Verification items for the finished model (mm, model axes). Face numbers are marked on the shaded views. A direction names the side the tool comes from. Give positions to 0.01 mm unless a question says otherwise; leave off trailing zeros. Write each loop counter-clockwise with the first axis right and the second up, starting at its lowest first coordinate (ties: lowest second). Pieces come first, ordered by that corner, then holes. Notation, with made-up numbers: M -15.5,15.25 L 17.5,15.25 A9 ccw 17.5,27.25 Z; hole C -24.5,62 d10. An arc over 180 degrees is marked long. Answer as a JSON object with one key per item and string values.
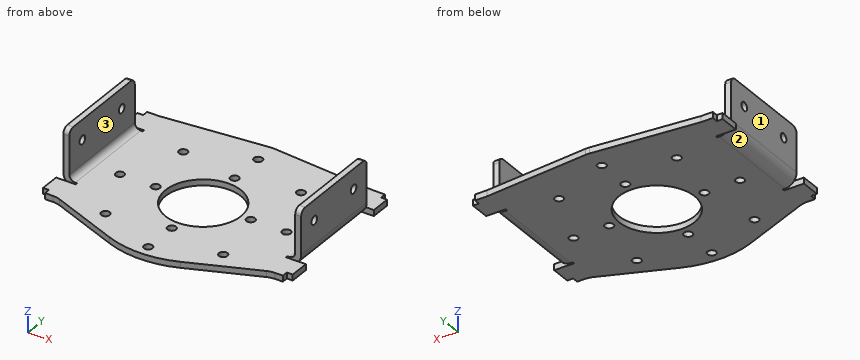
```python
from build123d import *

# Parameters (mm, degrees)
SKETCH1_R                = 19.05
SKETCH1_R_2              = 1
BASE_FLANGE1_DEPTH       = 3
UP_DEPTH                 = 50
UP_START                 = -3
UP_PROFILE_W             = 50
UP_PROFILE_H             = 22
UP_PROFILE_R             = 1
UP_FLAT_DEPTH            = 3
M4_CLEARANCE_HOLE1_D     = 4.3
M4_CLEARANCE_HOLE1_DEPTH = 136
M4_CLEARANCE_HOLE1_TIP   = 1.291850331
M4_CLEARANCE_HOLE2_D     = 4.3
M4_CLEARANCE_HOLE2_DEPTH = 136
M4_CLEARANCE_HOLE2_TIP   = 1.291850331
FILLET1_R                = 10
FILLET2_R                = 3


# Sheet-metal steps are written as plain solids
with BuildPart() as part:
    # Sketch1 → Base-Flange1 (new body)
    with BuildSketch(Plane.XY):
        with BuildLine():
            Line((-54, -30), (-17.930398419, -44.525282846))
            ThreePointArc((-17.930398419, -44.525282846), (0, -48), (17.930398419, -44.525282846))
            Line((17.930398419, -44.525282846), (54, -30))
            Line((54, -30), (60, -30))
            Line((60, -30), (60, -27))
            Line((60, -27), (63, -27))
            Line((63, -27), (63, -17))
            Line((63, -17), (53, -17))
            Line((53, -17), (53, -16))
            Line((53, -16), (54, -16))
            Line((54, -16), (54, 34))
            Line((54, 34), (53, 34))
            Line((53, 34), (53, 35))
            Line((53, 35), (63, 35))
            Line((63, 35), (63, 45))
            Line((63, 45), (60, 45))
            Line((60, 45), (60, 48))
            Line((60, 48), (54, 48))
            Line((54, 48), (0, 53))
            Line((0, 53), (-54, 48))
            Line((-54, 48), (-60, 48))
            Line((-60, 48), (-60, 45))
            Line((-60, 45), (-63, 45))
            Line((-63, 45), (-63, 35))
            Line((-63, 35), (-53, 35))
            Line((-53, 35), (-53, 34))
            Line((-53, 34), (-54, 34))
            Line((-54, 34), (-54, -16))
            Line((-54, -16), (-53, -16))
            Line((-53, -16), (-53, -17))
            Line((-53, -17), (-63, -17))
            Line((-63, -17), (-63, -27))
            Line((-63, -27), (-60, -27))
            Line((-60, -27), (-60, -30))
            Line((-60, -30), (-54, -30))
        make_face()
        Circle(SKETCH1_R, mode=Mode.SUBTRACT)
        with Locations((0, 24)):
            Circle(SKETCH1_R_2, mode=Mode.SUBTRACT)
        with Locations((0, -42)):
            Circle(SKETCH1_R_2, mode=Mode.SUBTRACT)
        with Locations((-29.69848481, -29.69848481)):
            Circle(SKETCH1_R_2, mode=Mode.SUBTRACT)
        with Locations((-42, 0)):
            Circle(SKETCH1_R_2, mode=Mode.SUBTRACT)
        with Locations((-29.69848481, 29.69848481)):
            Circle(SKETCH1_R_2, mode=Mode.SUBTRACT)
        with Locations((0, 42)):
            Circle(SKETCH1_R_2, mode=Mode.SUBTRACT)
        with Locations((29.69848481, 29.69848481)):
            Circle(SKETCH1_R_2, mode=Mode.SUBTRACT)
        with Locations((42, 0)):
            Circle(SKETCH1_R_2, mode=Mode.SUBTRACT)
        with Locations((29.69848481, -29.69848481)):
            Circle(SKETCH1_R_2, mode=Mode.SUBTRACT)
        with Locations((24, 0)):
            Circle(SKETCH1_R_2, mode=Mode.SUBTRACT)
        with Locations((0, -24)):
            Circle(SKETCH1_R_2, mode=Mode.SUBTRACT)
        with Locations((-24, 0)):
            Circle(SKETCH1_R_2, mode=Mode.SUBTRACT)
    extrude(amount=-BASE_FLANGE1_DEPTH)

    # UP bend section (across the edge) → UP (add)
    with BuildSketch(Plane(origin=(-57, 34, 0), x_dir=(1, 0, 0), z_dir=(0, -1, 0))):
        with BuildLine():
            Line((-3, 3), (0, 3))
            ThreePointArc((0, 3), (0.878679656, 0.878679656), (3, 0))
            Line((3, 0), (3, -3))
            ThreePointArc((3, -3), (-1.242640687, -1.242640687), (-3, 3))
        make_face()
    up = extrude(amount=UP_DEPTH)

    # UP profile (on flange) → UP flat (add)
    with BuildSketch(Plane.YZ.offset(-57).offset(UP_START)):
        with Locations((9, 14)):
            Rectangle(UP_PROFILE_W, UP_PROFILE_H)
        with Locations((-6, 15)):
            Circle(UP_PROFILE_R, mode=Mode.SUBTRACT)
        with Locations((24, 15)):
            Circle(UP_PROFILE_R, mode=Mode.SUBTRACT)
    up_flat = extrude(amount=UP_FLAT_DEPTH)

    # Mirror1: UP, UP flat across plane
    add(up.mirror(Plane(origin=(0, 0, 0), x_dir=(0, 0, 1), z_dir=(1, 0, 0))))
    add(up_flat.mirror(Plane(origin=(0, 0, 0), x_dir=(0, 0, 1), z_dir=(1, 0, 0))))

    # M4 Clearance Hole1
    with Locations(Plane.XY):
        with Locations((0, 24), (24, 0), (-24, 0), (0, -24), (0, -42), (29.69848481, -29.69848481), (42, 0), (29.69848481, 29.69848481), (0, 42), (-29.69848481, 29.69848481), (-42, 0), (-29.69848481, -29.69848481)):
            Hole(M4_CLEARANCE_HOLE1_D / 2, depth=M4_CLEARANCE_HOLE1_DEPTH)
            with Locations((0, 0, -(M4_CLEARANCE_HOLE1_DEPTH + M4_CLEARANCE_HOLE1_TIP / 2))):  # 118° drill point
                Cone(0, M4_CLEARANCE_HOLE1_D / 2, M4_CLEARANCE_HOLE1_TIP, mode=Mode.SUBTRACT)

    # M4 Clearance Hole2
    with Locations(Plane.ZY.offset(60)):
        with Locations((15, 24), (15, -6)):
            Hole(M4_CLEARANCE_HOLE2_D / 2, depth=M4_CLEARANCE_HOLE2_DEPTH)
            with Locations((0, 0, -(M4_CLEARANCE_HOLE2_DEPTH + M4_CLEARANCE_HOLE2_TIP / 2))):  # 118° drill point
                Cone(0, M4_CLEARANCE_HOLE2_D / 2, M4_CLEARANCE_HOLE2_TIP, mode=Mode.SUBTRACT)

    # Fillet1
    fillet1_edges = [part.edges().sort_by_distance(p)[0] for p in [
        (0, 53, -1.5),
        (54, -30, -1.5),
        (-54, -30, -1.5),
    ]]
    fillet(fillet1_edges, radius=FILLET1_R)

    # Fillet2
    fillet2_edges = [part.edges().sort_by_distance(p)[0] for p in [
        (-58.5, 34, 25),
        (-58.5, -16, 25),
        (58.5, -16, 25),
        (58.5, 34, 25),
    ]]
    fillet(fillet2_edges, radius=FILLET2_R)


solid = part.part
```
1) Thickness scan on L1, parallel to Y at x = -58.8, z = 15; L2, parallel to X at y = 19, z = 8; L3, parallel to Z at x = 15.5, y = 20. Record the ranges inside material, lowest first.
Completed:
{"L1": "y = -16 to -8.15, -3.85 to 21.85, 26.15 to 34", "L2": "x = -60 to -57, 57 to 60", "L3": "z = -3 to 0"}
2) Section check B-B on z = 15. Record the boundary of the cut face in (x, y).
Completed:
{"outline": "M -60,-16 L -57,-16 L -57,-8.15 L -60,-8.15 Z; M -60,-3.85 L -57,-3.85 L -57,21.85 L -60,21.85 Z; M -60,26.15 L -57,26.15 L -57,34 L -60,34 Z; M 57,-16 L 60,-16 L 60,-8.15 L 57,-8.15 Z; M 57,-3.85 L 60,-3.85 L 60,21.85 L 57,21.85 Z; M 57,26.15 L 60,26.15 L 60,34 L 57,34 Z"}
3) Access from +Z, -Z, +X, -X, +Y, -Y to the whole of each face (thin tool, end or side, straight path). Record for the marked faces 1, 2 and 3.
Completed:
{"face 1": "+Z, -Z, -X, +Y, -Y", "face 2": "-Z, -X", "face 3": "+Z, +Y, -Y"}
4) Section check C-C on y = 24. Record the boundary of the cut face in (x, z), and give its area (3 significant figures).
Completed:
{"outline": "M -60,3 A6 ccw -54,-3 L -2.15,-3 L -2.15,0 L -54,0 A3 cw -57,3 L -57,12.85 L -60,12.85 Z; M -60,17.15 L -57,17.15 L -57,25 L -60,25 Z; M 2.15,-3 L 54,-3 A6 ccw 60,3 L 60,12.85 L 57,12.85 L 57,3 A3 cw 54,0 L 2.15,0 Z; M 57,17.15 L 60,17.15 L 60,25 L 57,25 Z", "area": "460 mm2"}
5) Go/stop test with flat-tipped pins: pin 1 (0.5 mm diameter, centred on y = -16.5, z = -2, fed in from -X); pin 2 (0.9 mm diameter, centred on x = 58, z = -1.5, fed in from -Y); pin 3 (10 mm diameter, centred on y = -11.5, z = 10, fed in from -X); pin 4 (2.5 mm diameter, centred on y = -28, z = -1.5, fed in from -X). Record where each tip stops, or that it passes through.
Completed:
{"pin 1": "stops at x = -53", "pin 2": "stops at y = -30", "pin 3": "stops at x = -60", "pin 4": "stops at x = -63"}
6) Section check A-A on y = 0. Count the separate pieces of the cut face and the enclosed holes in it, and give its area (3 significant figures).
Completed:
{"separate pieces": "6", "enclosed holes": "0", "area": "333 mm2"}
7) Section check D-D on z = 7. Record the boundary of the cut face in (x, y).
Completed:
{"outline": "M -60,-16 L -57,-16 L -57,34 L -60,34 Z; M 57,-16 L 60,-16 L 60,34 L 57,34 Z"}
